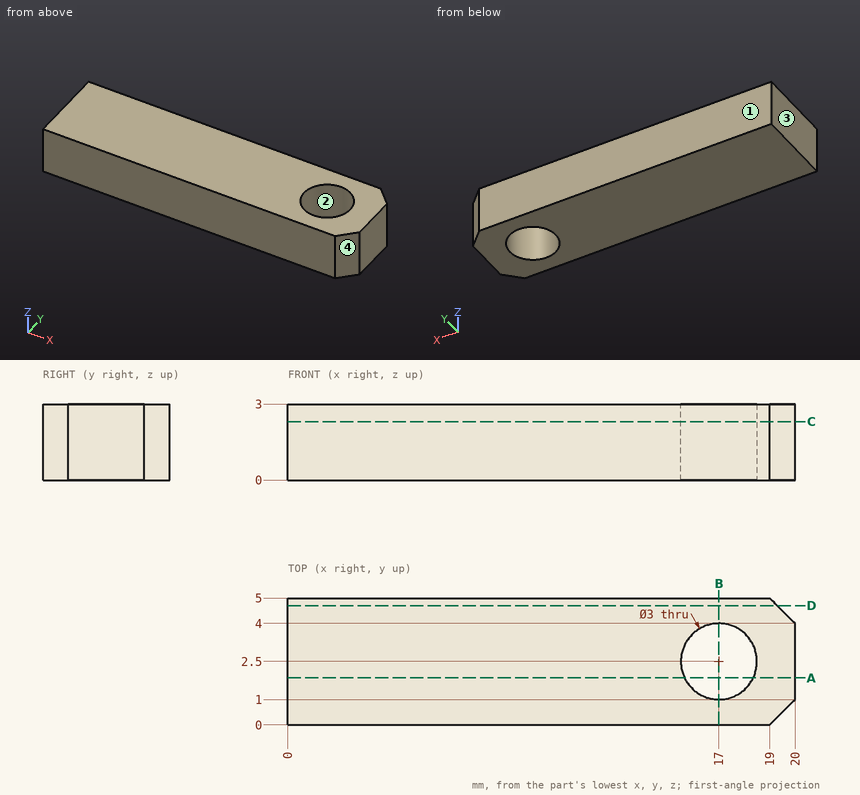
Verification items for this drawing (mm, ordinates from the low corner). Coordinates: 2 decimals unless noted, no trailing zeros. Write each loop counter-clockwise with the first axis right and the second up, starting at its lowest first coordinate (ties: lowest second). Pieces come first, ordered by that corner, then holes. Notation, with made-up numbers: (36, 50.25) -> (79, 50.25) arc R18 cw to (79, 70.25) -> close; hole circle Ø4 at (65, 51). An arc over 180 degrees is marked (long way). One line per item, written item: value. Start each with the question number.
Q1. Cross-section at C-C on z = 2.3. Enter the section's corners in (x, y).
Q2. Cross-section at B-B on x = 17. Enter the section's corners in (y, z), and give its area (3 significant figures).
Q3. Cross-section at D-D on y = 4.7. Enter the section's corners in (x, z), and give its area (3 significant figures).
Q4. Cross-section at A-A on y = 1.85. Enter the section's corners in (x, z).
Q5. Mould release check, pull along X, two halves, no side actions. Record for the marked faces 1, 2, 3 and 4: pulls with the +X half, pulls with the -X half, needs draft (parallel to the pull), parting line crosses it, or undercut.
Q6. Thickness scan on L1, parallel to Y at x = 17, z = 2.1; L2, parallel to X at y = 1.55, z = 2.5; L3, parallel to X at y = 1.4, z = 0.9. Record the ranges inside material, lowest first. Write a range as from..to.
Checked values:
1. outline: (0, 0) -> (19, 0) -> (20, 1) -> (20, 4) -> (19, 5) -> (0, 5) -> close; hole circle Ø3 at (17, 2.5)
2. outline: (0, 0) -> (1, 0) -> (1, 3) -> (0, 3) -> close; (4, 0) -> (5, 0) -> (5, 3) -> (4, 3) -> close
2. area: 6.00 mm²
3. outline: (0, 0) -> (19.3, 0) -> (19.3, 3) -> (0, 3) -> close
3. area: 57.9 mm²
4. outline: (0, 0) -> (15.65, 0) -> (15.65, 3) -> (0, 3) -> close; (18.35, 0) -> (20, 0) -> (20, 3) -> (18.35, 3) -> close
5. face 1: needs draft
5. face 2: undercut
5. face 3: pulls with the -X half
5. face 4: pulls with the +X half
6. L1: y = 0..1, 4..5
6. L2: x = 0..15.84, 18.16..20
6. L3: x = 0..15.98, 18.02..20
